Read the model definition and answer for the solid it produces. Units are mm, in the model's axes. A direction names the side the tool comes from. Coordinates: 2 decimals unless noted, no trailing zeros. Loops run counter-clockwise (first coordinate to the right, second up) from the corner with the lowest first, then second, coordinate; pieces in that order, holes last. Notation, with made-up numbers: (-21.75, 75.5) -> (11.25, 75.5) arc R16 ccw to (11.25, 106.5) -> close; hole circle Ø9 at (57.25, -7.75). An arc over 180 degrees is marked (long way). Answer in a Markdown table with one row per item.
```python
from build123d import *

# Parameters (mm, degrees)
SKETCH1_W                = 30
SKETCH1_H                = 32
BOSS_EXTRUDE1_DEPTH      = 14
CAVITY1_START            = 44.284378121
CAVITY1_OUTLINE_R        = 3
CAVITY1_DEPTH            = 32
M3_CLEARANCE_HOLE1_D     = 3
M3_CLEARANCE_HOLE1_DEPTH = 7
M3_CLEARANCE_HOLE1_TIP   = 0.901290929


# Read off the part's stored shape, not the designer's step: Cavity1
with BuildPart() as part:
    # Sketch1 → Boss-Extrude1 (new body)
    with BuildSketch(Plane(origin=(0, 8, 0), x_dir=(1, 0, 0), z_dir=(0, 1, 0))):
        with Locations((0, -60.284378121)):
            Rectangle(SKETCH1_W, SKETCH1_H)
    extrude(amount=-BOSS_EXTRUDE1_DEPTH)

    # Cavity1 outline → Cavity1 (cut)
    with BuildSketch(Plane.XY.offset(CAVITY1_START)):
        Circle(CAVITY1_OUTLINE_R)
    extrude(amount=CAVITY1_DEPTH, mode=Mode.SUBTRACT)

    # M3 Clearance Hole1
    with Locations(Plane(origin=(0, 8, 0), x_dir=(1, 0, 0), z_dir=(0, 1, 0))):
        with Locations((10.5, -49.784378121), (-10.5, -49.784378121), (-10.5, -70.784378121), (10.5, -70.784378121)):
            Hole(M3_CLEARANCE_HOLE1_D / 2, depth=M3_CLEARANCE_HOLE1_DEPTH)
            with Locations((0, 0, -(M3_CLEARANCE_HOLE1_DEPTH + M3_CLEARANCE_HOLE1_TIP / 2))):  # 118° drill point
                Cone(0, M3_CLEARANCE_HOLE1_D / 2, M3_CLEARANCE_HOLE1_TIP, mode=Mode.SUBTRACT)


solid = part.part
```
1. A cutting plane is placed at C-C on y = 5. Give the vertices of the cut face in (x, z), and give its area (3 significant figures).
A:
| item | result |
|---|---|
| outline | (-15, 44.28) -> (15, 44.28) -> (15, 76.28) -> (-15, 76.28) -> close; hole circle Ø3 at (-10.5, 49.78); hole circle Ø3 at (-10.5, 70.78); hole circle Ø3 at (10.5, 49.78); hole circle Ø3 at (10.5, 70.78) |
| area | 932 mm2 |
2. A tool of negligible diameter and unlimited length cuts with its end or side. For faces 4 (the cylindrical face through (11.606, 4.451, 48.771)), 5 (the flat face through (0, 8, 60)), from which of +Z, -Z, +X, -X, +Y, -Y can it reach the whole face along a straight path? Write none if from no direction.
A:
| item | result |
|---|---|
| face 4 | +Y |
| face 5 | +Z, -Z, +X, -X, +Y |
3. The mould has two halves that part along Y. Classify faces 1 (the cylindrical face through (-3, 0, 60)), 2 (the flat face through (0, 4, 44.284)), 3 (the conical face through (10.293, 0.255, 70.943)): pulls with the +Y half, pulls with the -Y half, needs draft (parallel to the pull), parting line crosses it, or undercut.
A:
| item | result |
|---|---|
| face 1 | undercut |
| face 2 | needs draft |
| face 3 | pulls with the +Y half |
4. A cutting plane is placed at B-B on x = 0. Give the vertices of the cut face in (y, z).
A:
| item | result |
|---|---|
| outline | (-6, 44.28) -> (-3, 44.28) -> (-3, 76.28) -> (-6, 76.28) -> close; (3, 44.28) -> (8, 44.28) -> (8, 76.28) -> (3, 76.28) -> close |
5. Find the intervals of material crossed by probe 1 along Z at (x, y) = (-10.5, 3); probe 2 along X at (y, z) = (5.25, 50); probe 3 along X at (y, z) = (2, 59), in increasing order.
A:
| item | result |
|---|---|
| probe 1 | z = 44.28 to 48.28, 51.28 to 69.28, 72.28 to 76.28 |
| probe 2 | x = -15 to -11.98, -9.02 to 9.02, 11.98 to 15 |
| probe 3 | x = -15 to -2.24, 2.24 to 15 |
6. A cutting plane is placed at A-A on z = 60.5. Give the vertices of the cut face in (x, y), and give its area (3 significant figures).
A:
| item | result |
|---|---|
| outline | (-15, -6) -> (15, -6) -> (15, 8) -> (-15, 8) -> close; hole circle Ø6 at (0, 0) |
| area | 392 mm2 |
